```python
from build123d import *

# Parameters (mm, degrees)
F1_DEPTH = 25.4
F2_R     = 2.19075
F3_DEPTH = 81.281
F4_R     = 5.3975
F5_DEPTH = 89.409


with BuildPart() as f1:
    # F0 (on Front) → F1 (new body)
    with BuildSketch(Plane.XZ):
        Polygon((25.908, -50.8), (38.608, -38.1), (63.5, -38.1), (63.5, 0), (0, 0), (-63.5, 0), (-63.5, -38.1), (-38.608, -38.1), (-25.908, -50.8), (-25.908, -81.28), (-13.208, -81.28), (-13.208, -12.7), (13.208, -12.7), (13.208, -81.28), (25.908, -81.28), align=None)
    extrude(amount=F1_DEPTH)

    # F2 (on face) → F3 (cut, through all)
    with BuildSketch(Plane.XY):
        with Locations((-44.45, -12.7)):
            Circle(F2_R)
        with Locations((44.45, -12.7)):
            Circle(F2_R)
    extrude(amount=-F3_DEPTH, mode=Mode.SUBTRACT)

    # F4 (on face) → F5 (cut, through all)
    with BuildSketch(Plane.YZ.offset(25.908)):
        with Locations((-12.7, -68.58)):
            Circle(F4_R)
    extrude(amount=-F5_DEPTH, mode=Mode.SUBTRACT)


solid = f1.part
```
CAD build for the part. Positions are in the model's coordinates, mm. A direction names the side the tool comes from. Coordinates: 2 decimals unless noted, no trailing zeros. Loops run counter-clockwise (first coordinate to the right, second up) from the corner with the lowest first, then second, coordinate; pieces in that order, holes last. Notation, with made-up numbers: (51.5, -14) - (68.5, -14) arc R36 cw to (68.5, 20) - close; hole circle Ø7 at (75.5, 15). An arc over 180 degrees is marked (long way). Return JSON: item names as keys, results as strings.
1. Band-saw the part on C-C (x = -44.45). Give the cut face in (y, z).
Result:
{"outline": "(-25.4, -38.1) - (-14.89, -38.1) - (-14.89, 0) - (-25.4, 0) - close; (-10.51, -38.1) - (0, -38.1) - (0, 0) - (-10.51, 0) - close"}
2. Drop flat-ended pins along their axis: pin 1 (12.5 mm diameter, centred on y = -12.7, z = -68.58, fed in from -X); pin 2 (12.5 mm diameter, centred on y = -17.5, z = -54.5, fed in from +X); pin 3 (6.5 mm diameter, centred on y = -12.7, z = -68.58, fed in from -X); pin 4 (5 mm diameter, centred on x = 32, y = -6.5, fed in from -Z). Give the stop position or say it passes through.
Result:
{"pin 1": "stops at x = -25.91", "pin 2": "stops at x = 28.46", "pin 3": "passes through", "pin 4": "stops at z = -47.21"}
3. Band-saw the part on D-D (z = -68.58). Give the cut face in (x, y), and give its area (3 significant figures).
Result:
{"outline": "(-25.91, -25.4) - (-13.21, -25.4) - (-13.21, -18.1) - (-25.91, -18.1) - close; (-25.91, -7.3) - (-13.21, -7.3) - (-13.21, 0) - (-25.91, 0) - close; (13.21, -25.4) - (25.91, -25.4) - (25.91, -18.1) - (13.21, -18.1) - close; (13.21, -7.3) - (25.91, -7.3) - (25.91, 0) - (13.21, 0) - close", "area": "371 mm2"}
4. Band-saw the part on A-A (z = -35.5). Give the cut face in (x, y), and give its area (3 significant figures).
Result:
{"outline": "(-63.5, -25.4) - (-13.21, -25.4) - (-13.21, 0) - (-63.5, 0) - close; (13.21, -25.4) - (63.5, -25.4) - (63.5, 0) - (13.21, 0) - close; hole circle Ø4.38 at (-44.45, -12.7); hole circle Ø4.38 at (44.45, -12.7)", "area": "2,520 mm2"}
5. 3-axis set-ups, long thin cutter, end or side, ignore diameter. For faces 1 (the flat face through (-15, -25.4, -31)), 2 (the flat face through (-51, -13, -38.1)), 3 (the flat face through (-13.208, -13, -47)), 4 (the flat face through (25.908, -13, -63)), 5 (the flat face through (-63.5, -13, -19)): which of +Z, -Z, +X, -X, +Y, -Y reach the whole face in a straight line?
Result:
{"face 1": "+Z, -Z, +X, -X, -Y", "face 2": "-Z, -X, +Y, -Y", "face 3": "-Z, +Y, -Y", "face 4": "-Z, +X, +Y, -Y", "face 5": "+Z, -Z, -X, +Y, -Y"}
6. Band-saw the part on B-B (y = -12.7). State how many separate pieces and enclosed holes the cut face has, and give its area (3 significant figures).
Result:
{"separate pieces": "5", "enclosed holes": "0", "area": "4,820 mm2"}
7. Probe L1, parallel to X at y = -16.25, z = -29.5; L2, parallel to X at y = -18.25, z = -75.5; L3, parallel to Z at x = 22.5, y = -13.25. List the from-to ranges inside material, lowest first. Write a range as from..to.
Result:
{"L1": "x = -63.5..-13.21, 13.21..63.5", "L2": "x = -25.91..-13.21, 13.21..25.91", "L3": "z = -81.28..-73.95, -63.21..0"}
8. Mould opens along X. For faces 6 (the flat face through (32.17, -12.52, -44.54)), 7 (the flat face through (51, -13, -38.1)), 8 (the flat face through (13.208, -13, -47)) say: released by +X, released by -X, zero draft, split by the parting line, or undercut.
Result:
{"face 6": "released by +X", "face 7": "zero draft", "face 8": "undercut"}
